from build123d import *

# Parameters (mm, degrees)
SKETCH_1_R      = 10.5
SKETCH_1_R_2    = 5.5
SKETCH_1_R_3    = 1.9
EXTRUDE_1_DEPTH = 3
SKETCH_1_3_R    = 5.5
EXTRUDE_2_DEPTH = 10


with BuildPart() as part:
    # Sketch 1 → Extrude 1 (new body)
    # profile 1 of 2: a face of its own
    with BuildSketch(Plane(origin=(0, 0, 0), x_dir=(1, 0, 0), z_dir=(0, 1, 0))):
        with Locations(Location((0, 0, 0), (0, 0, 270))):
            Circle(SKETCH_1_R)
        Circle(SKETCH_1_R_2, mode=Mode.SUBTRACT)
        with Locations(Location((0, 8, 0), (0, 0, 270))):
            Circle(SKETCH_1_R_3, mode=Mode.SUBTRACT)
        with Locations(Location((-8, 0, 0), (0, 0, 270))):
            Circle(SKETCH_1_R_3, mode=Mode.SUBTRACT)
        with Locations(Location((0, -8, 0), (0, 0, 270))):
            Circle(SKETCH_1_R_3, mode=Mode.SUBTRACT)
        with Locations(Location((8, 0, 0), (0, 0, 270))):
            Circle(SKETCH_1_R_3, mode=Mode.SUBTRACT)
    # profile 2 of 2: a face of its own
    with BuildSketch(Plane(origin=(0, 0, 0), x_dir=(1, 0, 0), z_dir=(0, 1, 0))):
        Circle(SKETCH_1_R_2)
    extrude(amount=EXTRUDE_1_DEPTH)

    # Sketch 1_3 → Extrude 2 (add)
    with BuildSketch(Plane(origin=(0, 0, 0), x_dir=(1, 0, 0), z_dir=(0, 1, 0))):
        with Locations(Location((0, 0, 0), (0, 0, 270))):
            Circle(SKETCH_1_3_R)
    extrude(amount=EXTRUDE_2_DEPTH)


solid = part.part
Input: part model. Units: mm. Frame: model coordinates. A direction names the side the tool comes from. Round coordinates to 2 decimals unless told otherwise and drop trailing zeros. Write each loop counter-clockwise with the first axis right and the second up, starting at its lowest first coordinate (ties: lowest second). Pieces come first, ordered by that corner, then holes.
1) Cut plane B-B (x = 0). Return the cut outline in (y, z), then the cut area to 3 significant figures.
2) Cut plane A-A (z = 0). Return the cut outline in (x, y), then the cut area to 3 significant figures.
3) Reachability of faces 1 (the flat face through (0, 0, 0)), 2 (the cylindrical face through (-5.37, 6.45, -1.19)) from +Z, -Z, +X, -X, +Y, -Y: full face, straight path, thin tool, end or side. Return the list, or none.
4) Ray query, L1, parallel to X at y = 0.6, z = 0; L2, parallel to Z at x = 1, y = 1.25; L3, parallel to Y at x = 1.5, z = -6. Return the intervals inside material, ascending.
5) Cut plane D-D (x = -8). Return the cut outline in (y, z).
6) Draft query along X for faces 3 (the cylindrical face through (-9.686, 1.479, 0.877)), 4 (the cylindrical face through (3.2, 1.5, 10)), 5 (the flat face through (-5, 3, 5)). Return one class per face: pulls with the +X half, pulls with the -X half, needs draft (parallel to the pull), parting line crosses it, or undercut.
7) Contact query for flat-ended pins moving along their axis: P1, Ø5, axis at x = 6.5, z = 5.5, coming from the +Y side; P2, Ø3, axis at y = 1, z = 4.5, coming from the +X side; P3, Ø2, axis at x = -3, y = 7, coming from the +Z side. Output: stop coordinate, or through.
8) Cut plane C-C (z = 8). Return the cut outline in (x, y).
Geometry says:
1. outline: (0, -10.5) - (3, -10.5) - (3, -9.9) - (0, -9.9) - close; (0, -6.1) - (3, -6.1) - (3, -5.5) - (10, -5.5) - (10, 5.5) - (3, 5.5) - (3, 6.1) - (0, 6.1) - close; (0, 9.9) - (3, 9.9) - (3, 10.5) - (0, 10.5) - close
1. area: 117 mm2
2. outline: (-10.5, 0) - (-9.9, 0) - (-9.9, 3) - (-10.5, 3) - close; (-6.1, 0) - (6.1, 0) - (6.1, 3) - (5.5, 3) - (5.5, 10) - (-5.5, 10) - (-5.5, 3) - (-6.1, 3) - close; (9.9, 0) - (10.5, 0) - (10.5, 3) - (9.9, 3) - close
2. area: 117 mm2
3. face 1: +Z, -Z, +X, -X, -Y
3. face 2: +Y
4. L1: x = -10.5 to -9.9, -6.1 to 6.1, 9.9 to 10.5
4. L2: z = -10.45 to -9.62, -6.38 to 6.38, 9.62 to 10.45
4. L3: y = 0 to 3
5. outline: (0, -6.8) - (3, -6.8) - (3, -1.9) - (0, -1.9) - close; (0, 1.9) - (3, 1.9) - (3, 6.8) - (0, 6.8) - close
6. face 3: undercut
6. face 4: parting line crosses it
6. face 5: needs draft
7. P1: stops at y = 3
7. P2: stops at x = 10.06
7. P3: stops at z = 5.12
8. outline: (-6.8, 0) - (-1.9, 0) - (-1.9, 3) - (-6.8, 3) - close; (1.9, 0) - (6.8, 0) - (6.8, 3) - (1.9, 3) - close
